```python
from build123d import *

# Parameters (mm, degrees)
F0_W     = 8.4663171785
F0_H     = 4.75
F1_DEPTH = 2.98


with BuildPart() as f1:
    # F0 (on Front) → F1 (new body)
    with BuildSketch(Plane.XZ):
        with Locations((14.7712850711, -37.7893784919)):
            Rectangle(F0_W, F0_H)
        with BuildLine():
            Line((19.7712850711, -8.4143784919), (19.7712850711, -5.4643784919))
            Line((19.7712850711, -5.4643784919), (9.7712850711, -5.4643784919))
            Line((9.7712850711, -5.4643784919), (9.7712850711, -8.4643784919))
            Line((9.7712850711, -8.4643784919), (-5.5287149289, -8.4643784919))
            ThreePointArc((-5.5287149289, -8.4643784919), (-9.0642488348, -9.9288445859), (-10.5287149289, -13.4643784919))
            Line((-10.5287149289, -13.4643784919), (-10.5287149289, -15.8643784919))
            Line((-10.5287149289, -15.8643784919), (-10.5287149289, -35.1643784919))
            ThreePointArc((-10.5287149289, -35.1643784919), (-9.0642488348, -38.6999123978), (-5.5287149289, -40.1643784919))
            Line((-5.5287149289, -40.1643784919), (10.5381264819, -40.1643784919))
            Line((10.5381264819, -40.1643784919), (10.5381264819, -35.4143784919))
            Line((10.5381264819, -35.4143784919), (-5.5287149289, -35.4143784919))
            ThreePointArc((-5.5287149289, -35.4143784919), (-5.7408469632, -35.3265105262), (-5.8287149289, -35.1143784919))
            Line((-5.8287149289, -35.1143784919), (-5.8287149289, -26.9643784919))
            Line((-5.8287149289, -26.9643784919), (-7.5287149289, -26.9643784919))
            ThreePointArc((-7.5287149289, -26.9643784919), (-8.2358217101, -26.6714852731), (-8.5287149289, -25.9643784919))
            Line((-8.5287149289, -25.9643784919), (-8.5287149289, -24.9643784919))
            ThreePointArc((-8.5287149289, -24.9643784919), (-8.2358217101, -24.2572717107), (-7.5287149289, -23.9643784919))
            Line((-7.5287149289, -23.9643784919), (-5.8287149289, -23.9643784919))
            Line((-5.8287149289, -23.9643784919), (-5.8287149289, -15.8143784919))
            ThreePointArc((-5.8287149289, -15.8143784919), (-5.7408469632, -15.6022464575), (-5.5287149289, -15.5143784919))
            Line((-5.5287149289, -15.5143784919), (35.0712850711, -15.5143784919))
            ThreePointArc((35.0712850711, -15.5143784919), (35.2834171055, -15.6022464575), (35.3712850711, -15.8143784919))
            Line((35.3712850711, -15.8143784919), (35.3712850711, -35.1143784919))
            ThreePointArc((35.3712850711, -35.1143784919), (35.2834171055, -35.3265105262), (35.0712850711, -35.4143784919))
            Line((35.0712850711, -35.4143784919), (19.0044436604, -35.4143784919))
            Line((19.0044436604, -35.4143784919), (19.0044436604, -40.1643784919))
            Line((19.0044436604, -40.1643784919), (35.0712850711, -40.1643784919))
            ThreePointArc((35.0712850711, -40.1643784919), (38.6068189771, -38.6999123978), (40.0712850711, -35.1643784919))
            Line((40.0712850711, -35.1643784919), (40.0712850711, -13.4143784919))
            ThreePointArc((40.0712850711, -13.4143784919), (38.6068189771, -9.8788445859), (35.0712850711, -8.4143784919))
            Line((35.0712850711, -8.4143784919), (19.7712850711, -8.4143784919))
        make_face()
    extrude(amount=F1_DEPTH)


solid = f1.part
```
Geometry: final body of the model. Coordinates: model frame, mm. A direction names the side the tool comes from. Coordinates: 2 decimals unless noted, no trailing zeros. Loops run counter-clockwise (first coordinate to the right, second up) from the corner with the lowest first, then second, coordinate; pieces in that order, holes last. Notation, with made-up numbers: (-9, 3) -> (33, 3) arc R34 cw to (33, 36) -> close; hole circle Ø3 at (32.25, 20.5). An arc over 180 degrees is marked (long way). Use a Markdown table: item, result. Add a question column.
(1) Line query: line 1 along X through (y, z) = (-2.55, -23); line 2 along Z through (x, y) = (26, -0.1); line 3 along Z through (x, y) = (12, -0.15). Output: solid intervals per line, ascending.
(2) Section query A-A, the plane x = -3. Return loops of the section in (y, z).
(3) Access query for faces 1 (the flat face through (9.771, -1, -7)), 2 (the flat face through (28, -1, -8.414)), 3 (the flat face through (14, -1, -15.514)), 4 (the flat face through (15, -1, -5.464)). Directions: +Z, -Z, +X, -X, +Y, -Y. A direction counts if a zero-diameter tool reaches every point of the face in a straight line with its end or side. Return the directions, or none.
(4) Section query C-C, the plane y = -1.1. Return loops of the section in (x, z).
(5) Section query B-B, the plane z = -18.5. Return loops of the section in (x, y), plus the area to 3 significant figures.
(6) Section query D-D, the plane x = 37.5. Return loops of the section in (y, z).
(7) Pin query (flat end, axial travel): pin 1 Ø0.5 at (x, y) = (-7, -2) entering from +Z; pin 2 Ø1.4 at (x, y) = (-6.5, -2) entering from -Z; pin 3 Ø1.5 at (x, y) = (0.5, -1) entering from +Z; pin 4 Ø8 at (x, z) = (29, -20) entering from -Y. Return the tip coordinate at first contact, or that it passes through.
Answer:
| question | item | result |
|---|---|---|
| 1 | line 1 | x = -10.53 to -5.83, 35.37 to 40.07 |
| 1 | line 2 | z = -40.16 to -35.41, -15.51 to -8.41 |
| 1 | line 3 | z = -40.16 to -35.41, -15.51 to -5.46 |
| 2 | outline | (-2.98, -40.16) -> (0, -40.16) -> (0, -35.41) -> (-2.98, -35.41) -> close; (-2.98, -15.51) -> (0, -15.51) -> (0, -8.46) -> (-2.98, -8.46) -> close |
| 3 | face 1 | +Z, -X, +Y, -Y |
| 3 | face 2 | +Z, +X, +Y, -Y |
| 3 | face 3 | +Y, -Y |
| 3 | face 4 | +Z, +X, -X, +Y, -Y |
| 4 | outline | (-10.53, -35.16) arc R5 ccw to (-5.53, -40.16) -> (35.07, -40.16) arc R5 ccw to (40.07, -35.16) -> (40.07, -13.41) arc R5 ccw to (35.07, -8.41) -> (19.77, -8.41) -> (19.77, -5.46) -> (9.77, -5.46) -> (9.77, -8.46) -> (-5.53, -8.46) arc R5 ccw to (-10.53, -13.46) -> close; hole (-8.53, -25.96) arc R1 ccw to (-7.53, -26.96) -> (-5.83, -26.96) -> (-5.83, -35.11) arc R0.3 ccw to (-5.53, -35.41) -> (35.07, -35.41) arc R0.3 ccw to (35.37, -35.11) -> (35.37, -15.81) arc R0.3 ccw to (35.07, -15.51) -> (-5.53, -15.51) arc R0.3 ccw to (-5.83, -15.81) -> (-5.83, -23.96) -> (-7.53, -23.96) arc R1 ccw to (-8.53, -24.96) -> close |
| 5 | outline | (-10.53, -2.98) -> (-5.83, -2.98) -> (-5.83, 0) -> (-10.53, 0) -> close; (35.37, -2.98) -> (40.07, -2.98) -> (40.07, 0) -> (35.37, 0) -> close |
| 5 | area | 28.0 mm^2 |
| 6 | outline | (-2.98, -39.53) -> (0, -39.53) -> (0, -9.04) -> (-2.98, -9.04) -> close |
| 7 | pin 1 | stops at z = -8.62 |
| 7 | pin 2 | stops at z = -40.16 |
| 7 | pin 3 | stops at z = -8.46 |
| 7 | pin 4 | passes through |
